Check sheet for the modelled part. Datum: model origin and axes. Units: mm. A direction names the side the tool comes from. Coordinates: 2 decimals unless noted, no trailing zeros. Write each loop counter-clockwise with the first axis right and the second up, starting at its lowest first coordinate (ties: lowest second). Pieces come first, ordered by that corner, then holes. Notation, with made-up numbers: M -20.5,21 L -11.5,21 A12 ccw -11.5,29 Z; hole C 22.25,21.25 d2. An arc over 180 degrees is marked long. Answer as CSV lines item,"result". Start each with the question number.
1) Section check A-A (x = -53). Record the cut outline in (y, z), and give its area (3 significant figures).
2) Access from +Z, -Z, +X, -X, +Y, -Y to the whole of each face (thin tool, end or side, straight path). Record for faces 1 (the flat face through (27, -43, 7.332)), 2 (the flat face through (-1, -63.5, 23)).
3) Material ranges on L1, parallel to X at y = 50.8, z = 21; L2, parallel to Y at x = -50.8, z = 14; L3, parallel to Z at x = 51.5, y = -49, recorded low to high. Write a range as [from, to].
4) Section check C-C (x = 0). Record the cut outline in (y, z).
5) Go/stop test with a flat-tipped pin: pin 1 Ø6 at (x, y) = (43, -43) entering from -Z. Record where the tip stops, or that it passes through.
6) Section check D-D (y = 0). Record the cut outline in (x, z).
7) Section check B-B (y = 55). Record the cut outline in (x, z).
from build123d import *

# Parameters (mm, degrees)
F1_W     = 127
F1_H     = 38.1
F2_DEPTH = 63.5
F5_DEPTH = 50.8


with BuildPart() as f2:
    # F1 (on Front) → F2 (new body, symmetric)
    with BuildSketch(Plane.XZ):
        with Locations((-0.005746, 19.05)):
            Rectangle(F1_W, F1_H)
    extrude(amount=F2_DEPTH, both=True)

    # F0 (on Front) → F3 (revolve, cut)
    with BuildSketch(Plane.XZ):
        Polygon((48.160355, 7.332348), (38.1, 1.524), (0, 1.524), (0, 0), (92.567263, 0), (92.567263, 7.332348), align=None)
    revolve(axis=Axis((0, 0, 0.762), (0, 0, -1)), mode=Mode.SUBTRACT)

    # F4 (on Top) → F5 (cut, symmetric)
    with BuildSketch(Plane.XY):
        with BuildLine():
            Line((-50.8, 44.45), (-50.8, 50.8))
            Line((-50.8, 50.8), (-44.45, 50.8))
            ThreePointArc((-44.45, 50.8), (-55.290128, 55.290128), (-50.8, 44.45))
        make_face()
        with BuildLine():
            Line((-44.45, 50.8), (-50.8, 50.8))
            Line((-50.8, 50.8), (-50.8, 44.45))
            ThreePointArc((-50.8, 44.45), (-46.309872, 46.309872), (-44.45, 50.8))
        make_face()
    extrude(amount=F5_DEPTH, both=True, mode=Mode.SUBTRACT)


solid = f2.part
Results found:
1,outline,"M -63.5,7.33 L 44.84,7.33 L 44.84,38.1 L -63.5,38.1 Z; M 56.76,7.33 L 63.5,7.33 L 63.5,38.1 L 56.76,38.1 Z"
1,area,"3,540 mm2"
2,face 1,"-Z"
2,face 2,"+Z, -Z, +X, -X, -Y"
3,L1,"x = [-63.51, -57.15], [-44.45, 63.49]"
3,L2,"y = [-63.5, 44.45], [57.15, 63.5]"
3,L3,"z = [7.33, 38.1]"
4,outline,"M -63.5,7.33 L -48.16,7.33 L -38.1,1.52 L 38.1,1.52 L 48.16,7.33 L 63.5,7.33 L 63.5,38.1 L -63.5,38.1 Z"
5,pin 1,"stops at z = 7.33"
6,outline,"M -63.51,7.33 L -48.16,7.33 L -38.1,1.52 L 38.1,1.52 L 48.16,7.33 L 63.49,7.33 L 63.49,38.1 L -63.51,38.1 Z"
7,outline,"M -63.51,7.33 L -55.56,7.33 L -55.56,38.1 L -63.51,38.1 Z; M -46.04,7.33 L 63.49,7.33 L 63.49,38.1 L -46.04,38.1 Z"
